Input: part model. Units: mm. Frame: model coordinates. Face numbers are marked on the shaded views. A direction names the side the tool comes from. Coordinates: 2 decimals unless noted, no trailing zeros. Write each loop counter-clockwise with the first axis right and the second up, starting at its lowest first coordinate (ties: lowest second). Pieces come first, ordered by that corner, then holes. Notation, with made-up numbers: (85, 44) - (134, 44) arc R15 ccw to (134, 61) - close; hole circle Ø4 at (48, -11.75). An arc over 180 degrees is marked (long way). Use CSV: the item, a comma, the result in double quotes.
```python
from build123d import *

# Parameters (mm, degrees)
F0_R     = 4.25
F0_R_2   = 2.25
F1_DEPTH = 4
F0_R_3   = 8
F0_R_4   = 5
F2_DEPTH = 1.5


with BuildPart() as f1:
    # F0 (on Right) → F1 (new body)
    with BuildSketch(Plane.YZ):
        with Locations((-5.2978091688, 6.2685288617)):
            Circle(F0_R)
        with Locations((-5.2978091688, 6.2685288617)):
            Circle(F0_R_2, mode=Mode.SUBTRACT)
    extrude(amount=F1_DEPTH)

    # F0 (on Right) → F2 (join)
    with BuildSketch(Plane.YZ):
        with Locations((-5.2978091688, 6.2685288617)):
            Circle(F0_R_3)
        with Locations((-5.2978091688, 6.2685288617)):
            Circle(F0_R_4, mode=Mode.SUBTRACT)
        with Locations((-5.2978091688, 6.2685288617)):
            Circle(F0_R_4)
        with Locations((-5.2978091688, 6.2685288617)):
            Circle(F0_R, mode=Mode.SUBTRACT)
        with Locations((-5.2978091688, 6.2685288617)):
            Circle(F0_R)
        with Locations((-5.2978091688, 6.2685288617)):
            Circle(F0_R_2, mode=Mode.SUBTRACT)
    extrude(amount=-F2_DEPTH)


solid = f1.part
```
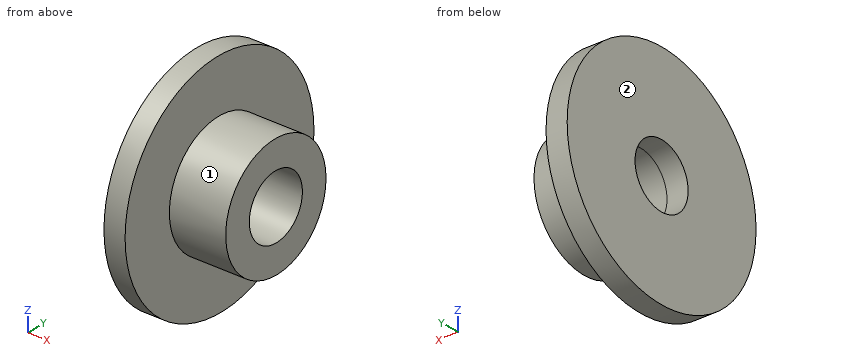
(1) Cut plane B-B on y = -4.75. Return loops of the section in (x, z), and give its area (3 significant figures).
Check values:
outline,"(-1.5, -1.71) - (0, -1.71) - (0, 2.05) - (4, 2.05) - (4, 4.09) - (-1.5, 4.09) - close; (-1.5, 8.45) - (4, 8.45) - (4, 10.48) - (0, 10.48) - (0, 14.25) - (-1.5, 14.25) - close"
area,"33.7 mm^2"
(2) Reachability of the marked faces 1 and 2 from +Z, -Z, +X, -X, +Y, -Y: full face, straight path, thin tool, end or side. Return the list, or none.
Check values:
face 1,"+X"
face 2,"+Z, -Z, -X, +Y, -Y"
(3) Cut plane D-D on x = 3.2. Return loops of the section in (y, z).
Check values:
outline,"circle Ø8.5 at (-5.3, 6.27); hole circle Ø4.5 at (-5.3, 6.27)"
(4) Pin query (flat end, axial travel): pin 1 Ø1.5 at (x, y) = (2.5, -9.5) entering from +Z; pin 2 Ø2.5 at (y, z) = (-5.3, 6.27) entering from +X; pin 3 Ø3 at (y, z) = (-11, 0.5) entering from +X. Return the tip coordinate at first contact, or that it passes through.
Check values:
pin 1,"z = 8.75"
pin 2,"through"
pin 3,"x = 0"
(5) Ray query, probe 1 along X at (y, z) = (1.5, 9); probe 2 along Y at (x, z) = (3.2, 8); probe 3 along Z at (x, y) = (3, -4.75). Return the intervals inside material, ascending. Write a range as from..to.
Check values:
probe 1,"-1.5..0"
probe 2,"-9.18..-6.73, -3.86..-1.42"
probe 3,"2.05..4.09, 8.45..10.48"
(6) Cut plane C-C on y = -8. Return loops of the section in (x, z), and give its area (3 significant figures).
Check values:
outline,"(-1.5, -1.26) - (0, -1.26) - (0, 2.99) - (4, 2.99) - (4, 9.55) - (0, 9.55) - (0, 13.8) - (-1.5, 13.8) - close"
area,"48.8 mm^2"
(7) Cut plane A-A on z = 5.75. Return loops of the section in (x, y).
Check values:
outline,"(-1.5, -13.28) - (0, -13.28) - (0, -9.52) - (4, -9.52) - (4, -7.49) - (-1.5, -7.49) - close; (-1.5, -3.11) - (4, -3.11) - (4, -1.08) - (0, -1.08) - (0, 2.69) - (-1.5, 2.69) - close"
